from build123d import *

# Parameters (mm, degrees)
SKETCH1_W   = 35
SKETCH1_H   = 20
PCB_DEPTH   = 1.6
HOLES_REACH = 22.219
SKETCH2_R   = 1.15


with BuildPart() as part:
    # Sketch1 → PCB (new body)
    with BuildSketch(Plane.XY):
        Rectangle(SKETCH1_W, SKETCH1_H)
    extrude(amount=PCB_DEPTH)

    # Sketch2 → Holes (cut, up to next)
    with BuildSketch(Plane.XY, mode=Mode.PRIVATE) as holes_sk1:
        with Locations((12.5, 7)):
            Circle(SKETCH2_R)
    holes_tool1 = extrude(holes_sk1.sketch, amount=HOLES_REACH, mode=Mode.PRIVATE) & part.part
    # Sketch2 → Holes (cut, up to next)
    with BuildSketch(Plane.XY, mode=Mode.PRIVATE) as holes_sk2:
        with Locations((-6.5, 7)):
            Circle(SKETCH2_R)
    holes_tool2 = extrude(holes_sk2.sketch, amount=HOLES_REACH, mode=Mode.PRIVATE) & part.part
    # Sketch2 → Holes (cut, up to next)
    with BuildSketch(Plane.XY, mode=Mode.PRIVATE) as holes_sk3:
        with Locations((-6.5, -7)):
            Circle(SKETCH2_R)
    holes_tool3 = extrude(holes_sk3.sketch, amount=HOLES_REACH, mode=Mode.PRIVATE) & part.part
    # Sketch2 → Holes (cut, up to next)
    with BuildSketch(Plane.XY, mode=Mode.PRIVATE) as holes_sk4:
        with Locations((12.5, -7)):
            Circle(SKETCH2_R)
    holes_tool4 = extrude(holes_sk4.sketch, amount=HOLES_REACH, mode=Mode.PRIVATE) & part.part
    add(holes_tool1.solids().sort_by_distance((12.5, 7, 0))[0], mode=Mode.SUBTRACT)
    add(holes_tool2.solids().sort_by_distance((-6.5, 7, 0))[0], mode=Mode.SUBTRACT)
    add(holes_tool3.solids().sort_by_distance((-6.5, -7, 0))[0], mode=Mode.SUBTRACT)
    add(holes_tool4.solids().sort_by_distance((12.5, -7, 0))[0], mode=Mode.SUBTRACT)


solid = part.part
For this review, take the finished solid that the model builds, in its own axes (mm). Round coordinates to 2 decimals unless told otherwise and drop trailing zeros. Write each loop counter-clockwise with the first axis right and the second up, starting at its lowest first coordinate (ties: lowest second). Pieces come first, ordered by that corner, then holes. Notation, with made-up numbers: M 23,61.5 L 47,61.5 A14 cw 47,68.5 Z; hole C 8,89 d6. An arc over 180 degrees is marked long. Write item = value, one per line. Start each with the question number.
(1) We need section A-A (x = 12.5). Give the boundary of the cut face in (y, z).
(2) The part is to be moulded in two halves that separate along X. For faces 1 (the face through (0, 10, 1)), 2 (the face through (-17.5, 0, 1)), 3 (the face through (13.12, -6.03, 0.79)), 4 (the face through (17.5, 0, 1)), say which applies: +X half, -X half, draft (parallel to the pull), parting line (faces both ways), or undercut.
(3) We need section C-C (z = 0.7). Give the boundary of the cut face in (x, y), then the cut area to 3 significant figures.
(4) Clearance check with flat-ended pins moving along their axes: pin 1 Ø3 at (x, y) = (12.5, 7) entering from +Z; pin 2 Ø2 at (x, y) = (-6.5, -7) entering from +Z. State where each tip first meets the part, or that it passes through.
(5) For line 1 along Y through (x, z) = (-6.5, 0.4); line 2 along X through (y, z) = (7, 0.7); line 3 along Y through (x, z) = (13, 0.3), list the stretches that pass through material, from the lowest coordinate up.
(6) We need section B-B (y = -7). Give the boundary of the cut face in (x, z), then the cut area to 3 significant figures.
Results found:
q1.outline = M -10,0 L -8.15,0 L -8.15,1.6 L -10,1.6 Z; M -5.85,0 L 5.85,0 L 5.85,1.6 L -5.85,1.6 Z; M 8.15,0 L 10,0 L 10,1.6 L 8.15,1.6 Z
q2.face_1 = draft
q2.face_2 = -X half
q2.face_3 = undercut
q2.face_4 = +X half
q3.outline = M -17.5,-10 L 17.5,-10 L 17.5,10 L -17.5,10 Z; hole C -6.5,-7 d2.3; hole C -6.5,7 d2.3; hole C 12.5,-7 d2.3; hole C 12.5,7 d2.3
q3.area = 683 mm²
q4.pin_1 = 1.6
q4.pin_2 = through
q5.line_1 = -10 to -8.15, -5.85 to 5.85, 8.15 to 10
q5.line_2 = -17.5 to -7.65, -5.35 to 11.35, 13.65 to 17.5
q5.line_3 = -10 to -8.04, -5.96 to 5.96, 8.04 to 10
q6.outline = M -17.5,0 L -7.65,0 L -7.65,1.6 L -17.5,1.6 Z; M -5.35,0 L 11.35,0 L 11.35,1.6 L -5.35,1.6 Z; M 13.65,0 L 17.5,0 L 17.5,1.6 L 13.65,1.6 Z
q6.area = 48.6 mm²
